from build123d import *

# Parameters (mm, degrees)
SKETCH_1_R          = 22.5
SKETCH_1_R_2        = 11.5
EXTRUDE_1_DEPTH     = 47
EXTRUDE_2_DEPTH     = 47
EXTRUDE_3_DEPTH     = 11
EXTRUDE_10_DEPTH    = 29
EXTRUDE_11_DEPTH    = 14
CUT_EXTRUDE_1_DEPTH = 138


with BuildPart() as part:
    # Sketch 1 → Extrude 1 (new body)
    with BuildSketch(Plane.XY):
        Circle(SKETCH_1_R)
        Circle(SKETCH_1_R_2, mode=Mode.SUBTRACT)
    extrude(amount=EXTRUDE_1_DEPTH)



with BuildPart() as body_2:
    # Sketch 3 → Extrude 2 (new body)
    with BuildSketch(Plane.XY.offset(9)):
        Polygon((-83, -68), (0, -68), (7, -68), (7, -54), (-83, -54), align=None)
    extrude(amount=EXTRUDE_2_DEPTH)


with BuildPart() as part_1:
    add(part.part)

    add(body_2.part)  # Extrude 3 merges body 2
    # Sketch 4 → Extrude 3 (add)
    with BuildSketch(Plane.XY.offset(9)):
        with BuildLine():
            Line((-83, -54), (-16.234704276, 15.578330368))
            ThreePointArc((-16.234704276, 15.578330368), (-21.829002199, -5.453866793), (-7, -21.38340478))
            Line((-7, -21.38340478), (-7, -54))
            Line((-7, -54), (-83, -54))
        make_face()
    extrude(amount=EXTRUDE_3_DEPTH)

    # Sketch 6 → Extrude 10 (add)
    with BuildSketch(Plane.XY.offset(9)):
        with BuildLine():
            Line((-7, -21.38340478), (-7, -54))
            Line((-7, -54), (7, -54))
            Line((7, -54), (7, -21.38340478))
            ThreePointArc((7, -21.38340478), (0, -22.5), (-7, -21.38340478))
        make_face()
    extrude(amount=EXTRUDE_10_DEPTH)

    # Sketch 7 → Extrude 11 (add)
    with BuildSketch(Plane(origin=(7, 0, 0), x_dir=(0, 0, -1), z_dir=(1, 0, 0))):
        Polygon((-38, -54), (-38, -40), (-56, -54), align=None)
    extrude(amount=-EXTRUDE_11_DEPTH)

    # Sketch 8 → Cut-Extrude 1 (cut)
    with BuildSketch(Plane(origin=(0, -168, 0), x_dir=(-1, 0, 0), z_dir=(0, -1, 0))):
        with BuildLine():
            Line((60, -45), (35, -45))
            ThreePointArc((35, -45), (28, -38), (35, -31))
            Line((35, -31), (60, -31))
            ThreePointArc((60, -31), (67, -38), (60, -45))
        make_face()
    extrude(amount=-CUT_EXTRUDE_1_DEPTH, mode=Mode.SUBTRACT)


solid = part_1.part
Read the model definition and answer for the solid it produces. Units are mm, in the model's axes. A direction names the side the tool comes from. Give positions to 0.01 mm unless a question says otherwise; leave off trailing zeros. Loops run counter-clockwise (first coordinate to the right, second up) from the corner with the lowest first, then second, coordinate; pieces in that order, holes last. Notation, with made-up numbers: (32, 77) -> (73, 77) arc R22 cw to (73, 111) -> close; hole circle Ø6 at (26.25, 39.5). An arc over 180 degrees is marked (long way). Use a Markdown table: item, result.
Q1. Each of these flat-tipped pins is pushed along its axis until it touches: pin 1 (4 mm diameter, centred on x = -2.5, y = -31.5, fed in from +Z); pin 2 (10 mm diameter, centred on y = -49.5, z = 8, fed in from +X); pin 3 (1.5 mm diameter, centred on y = -23, z = 30, fed in from -X). Where does it stop, or does it pass through?
Solved:
| item | result |
|---|---|
| pin 1 | stops at z = 38 |
| pin 2 | stops at x = 7 |
| pin 3 | stops at x = -7 |
Q2. Section A-A, the plane x = 0 is taken. Determine the outline of the cut face in (y, z).
Solved:
| item | result |
|---|---|
| outline | (-68, 9) -> (-22.5, 9) -> (-22.5, 0) -> (-11.5, 0) -> (-11.5, 47) -> (-22.5, 47) -> (-22.5, 38) -> (-40, 38) -> (-54, 56) -> (-68, 56) -> close; (11.5, 0) -> (22.5, 0) -> (22.5, 47) -> (11.5, 47) -> close |
Q3. Determine the mould class of faces 1 (the face through (-50.085, -19.698, 14.423)), 2 (the face through (-67, -61, 38)), 3 (the face through (-36, -34, 20)) for opening direction X: pulls with the +X half, pulls with the -X half, needs draft (parallel to the pull), parting line crosses it, or undercut.
Solved:
| item | result |
|---|---|
| face 1 | pulls with the -X half |
| face 2 | undercut |
| face 3 | needs draft |
Q4. Find the intervals of material crossed by line 1 along Z through (x, y) = (-59, -63); line 2 along Y through (x, z) = (0, 21); line 3 along Z through (x, y) = (-41.5, -39.5), in increasing order.
Solved:
| item | result |
|---|---|
| line 1 | z = 9 to 31, 45 to 56 |
| line 2 | y = -68 to -11.5, 11.5 to 22.5 |
| line 3 | z = 9 to 20 |
Q5. Section D-D, the plane y = 9.5 is taken. Determine the outline of the cut face in (x, z).
Solved:
| item | result |
|---|---|
| outline | (-22.07, 9) -> (-20.4, 9) -> (-20.4, 0) -> (-6.48, 0) -> (-6.48, 47) -> (-20.4, 47) -> (-20.4, 20) -> (-22.07, 20) -> close; (6.48, 0) -> (20.4, 0) -> (20.4, 47) -> (6.48, 47) -> close |
Q6. Section B-B, the plane y = -59 is taken. Determine the outline of the cut face in (x, z).
Solved:
| item | result |
|---|---|
| outline | (-83, 9) -> (7, 9) -> (7, 56) -> (-83, 56) -> close; hole (-60, 31) -> (-35, 31) arc R7 ccw to (-35, 45) -> (-60, 45) arc R7 ccw to start |
Q7. A tool of negligible diameter and unlimited length cuts with its end or side. For faces 4 (the face through (-48, -61, 45)), 5 (the face through (10, -10, 47)), 6 (the face through (-7, -41, 30)), 7 (the face through (-39, -61, 56)), 8 (the face through (0, -47, 47)), from which of +Z, -Z, +X, -X, +Y, -Y can it reach the whole face along a straight path? Write none if from no direction.
Solved:
| item | result |
|---|---|
| face 4 | +Y, -Y |
| face 5 | +Z, +X, -X, +Y |
| face 6 | +Z, -X |
| face 7 | +Z, +X, -X, +Y, -Y |
| face 8 | +Z, +X, -X |
Q8. Section C-C, the plane z = 14.5 is taken. Determine the outline of the cut face in (x, y).
Solved:
| item | result |
|---|---|
| outline | (-83, -68) -> (7, -68) -> (7, -21.38) arc R22.5 ccw (long way) to (-16.23, 15.58) -> (-83, -54) -> close; hole circle Ø23 at (0, 0) |
